Geometry: final body of the model. Coordinates: model frame, mm. Face numbers are marked on the shaded views. A direction names the side the tool comes from. Coordinates: 2 decimals unless noted, no trailing zeros. Loops run counter-clockwise (first coordinate to the right, second up) from the corner with the lowest first, then second, coordinate; pieces in that order, holes last. Notation, with made-up numbers: (-20.75, -33) -> (2.25, -33) arc R21 cw to (2.25, -11) -> close; hole circle Ø2 at (52.25, 50.5). An arc over 180 degrees is marked (long way). One line per item, written item: value. Start each with the question number.
from build123d import *

# Parameters (mm, degrees)
BOSS_EXTRUDE1_DEPTH     = 9
SKETCH2_W               = 152.4
SKETCH2_H               = 121
BOSS_EXTRUDE2_DEPTH     = 65
CHAMFER1_SIZE           = 10
SKETCH3_W               = 53.3
SKETCH3_H               = 12.5
CUT_EXTRUDE1_DEPTH      = 170.573612334
SKETCH4_R               = 2.5
BOSS_EXTRUDE3_DEPTH     = 1.780724539
CUT_EXTRUDE4_DEPTH      = 3
CUT_EXTRUDE4_DEPTH_BACK = 3
SKETCH5_R               = 1.5
CUT_EXTRUDE6_DEPTH      = 3
CUT_EXTRUDE6_DEPTH_BACK = 3
SKETCH7_W               = 9
SKETCH7_H               = 16.5
SKETCH8_R               = 8.25
CUT_EXTRUDE7_DEPTH      = 3
SKETCH9_R               = 1.5
CUT_EXTRUDE8_DEPTH      = 20


with BuildPart() as part:
    # Sketch1 → Boss-Extrude1 (new body)
    with BuildSketch(Plane(origin=(0, 0, 0), x_dir=(1, 0, 0), z_dir=(0, 1, 0))):
        with BuildLine():
            Line((-76.2, 63.5), (76.2, 63.5))
            ThreePointArc((76.2, 63.5), (85.180256121, 59.780256121), (88.9, 50.8))
            Line((88.9, 50.8), (88.9, -50.8))
            ThreePointArc((88.9, -50.8), (85.180256121, -59.780256121), (76.2, -63.5))
            Line((76.2, -63.5), (-76.2, -63.5))
            ThreePointArc((-76.2, -63.5), (-85.180256121, -59.780256121), (-88.9, -50.8))
            Line((-88.9, -50.8), (-88.9, 50.8))
            ThreePointArc((-88.9, 50.8), (-85.180256121, 59.780256121), (-76.2, 63.5))
        make_face()
    extrude(amount=BOSS_EXTRUDE1_DEPTH)

    # Sketch2 → Boss-Extrude2 (add)
    with BuildSketch(Plane(origin=(0, 9, 0), x_dir=(1, 0, 0), z_dir=(0, 1, 0))):
        with BuildLine():
            Line((76.2, 63.5), (-76.2, 63.5))
            ThreePointArc((-76.2, 63.5), (-85.180256121, 59.780256121), (-88.9, 50.8))
            Line((-88.9, 50.8), (-88.9, -50.8))
            ThreePointArc((-88.9, -50.8), (-85.180256121, -59.780256121), (-76.2, -63.5))
            Line((-76.2, -63.5), (76.2, -63.5))
            ThreePointArc((76.2, -63.5), (85.180256121, -59.780256121), (88.9, -50.8))
            Line((88.9, -50.8), (88.9, 50.8))
            ThreePointArc((88.9, 50.8), (85.180256121, 59.780256121), (76.2, 63.5))
        make_face()
        Rectangle(SKETCH2_W, SKETCH2_H, mode=Mode.SUBTRACT)
    extrude(amount=BOSS_EXTRUDE2_DEPTH)

    # Chamfer1
    chamfer1_edges = [part.edges().sort_by_distance(p)[0] for p in [
        (76.2, 41.5, -60.5),
        (-76.2, 41.5, -60.5),
        (-76.2, 41.5, 60.5),
        (76.2, 41.5, 60.5),
    ]]
    chamfer(chamfer1_edges, length=CHAMFER1_SIZE)

    # Sketch3 → Cut-Extrude1 (cut, through all)
    with BuildSketch(Plane.XY.offset(-60.5)):
        with Locations((-31.872362203, 17.030724539)):
            Rectangle(SKETCH3_W, SKETCH3_H)
    extrude(amount=-CUT_EXTRUDE1_DEPTH, mode=Mode.SUBTRACT)

    # Sketch4 → Boss-Extrude3 (add)
    with BuildSketch(Plane(origin=(0, 9, 0), x_dir=(1, 0, 0), z_dir=(0, 1, 0))):
        with Locations(Location((-56.511501143, 46.5, 0), (0, 0, 90))):
            Circle(SKETCH4_R)
        with Locations(Location((-8.211501143, 45.2, 0), (0, 0, 90))):
            Circle(SKETCH4_R)
        with Locations(Location((-23.411501143, -5.6, 0), (0, 0, 90))):
            Circle(SKETCH4_R)
        with Locations(Location((-51.311501143, -5.6, 0), (0, 0, 90))):
            Circle(SKETCH4_R)
    extrude(amount=BOSS_EXTRUDE3_DEPTH)

    # Sketch5 → Cut-Extrude4 (cut, two sides: drawn at the far end of the back side and taken through both)
    with BuildSketch(Plane(origin=(0, 10.780724539, 0), x_dir=(1, 0, 0), z_dir=(0, 1, 0)).offset(-CUT_EXTRUDE4_DEPTH_BACK)):
        with Locations(Location((-23.411501143, -5.6, 0), (0, 0, 270))):
            Circle(SKETCH5_R)
        with Locations(Location((-51.311501143, -5.6, 0), (0, 0, 270))):
            Circle(SKETCH5_R)
        with Locations(Location((-56.511501143, 46.5, 0), (0, 0, 270))):
            Circle(SKETCH5_R)
        with Locations(Location((-8.211501143, 45.2, 0), (0, 0, 270))):
            Circle(SKETCH5_R)
    extrude(amount=CUT_EXTRUDE4_DEPTH + CUT_EXTRUDE4_DEPTH_BACK, mode=Mode.SUBTRACT)

    # Sketch7 → Cut-Extrude6 (cut, two sides: drawn at the far end of the back side and taken through both)
    with BuildSketch(Plane.XY.offset(-60.5).offset(-CUT_EXTRUDE6_DEPTH_BACK)):
        with Locations((2.277637797, 19.030724539)):
            Rectangle(SKETCH7_W, SKETCH7_H)
    extrude(amount=CUT_EXTRUDE6_DEPTH + CUT_EXTRUDE6_DEPTH_BACK, mode=Mode.SUBTRACT)

    # Sketch8 → Cut-Extrude7 (cut)
    with BuildSketch(Plane.XY.offset(63.5)):
        with Locations((0, 37)):
            Circle(SKETCH8_R)
    extrude(amount=-CUT_EXTRUDE7_DEPTH, mode=Mode.SUBTRACT)

    # Sketch9 → Cut-Extrude8 (cut)
    with BuildSketch(Plane(origin=(0, 74, 0), x_dir=(1, 0, 0), z_dir=(0, 1, 0))):
        with Locations(Location((-80.555777772, -55.155777772, 0), (0, 0, 270))):
            Circle(SKETCH9_R)
        with Locations(Location((-80.555777772, 55.155777772, 0), (0, 0, 90))):
            Circle(SKETCH9_R)
        with Locations((29.755777772, -55.155777772)):
            Circle(SKETCH9_R)
        with Locations(Location((80.555777772, 55.155777772, 0), (0, 0, 270))):
            Circle(SKETCH9_R)
        with Locations(Location((80.555777772, -55.155777772, 0), (0, 0, 90))):
            Circle(SKETCH9_R)
    extrude(amount=-CUT_EXTRUDE8_DEPTH, mode=Mode.SUBTRACT)


solid = part.part
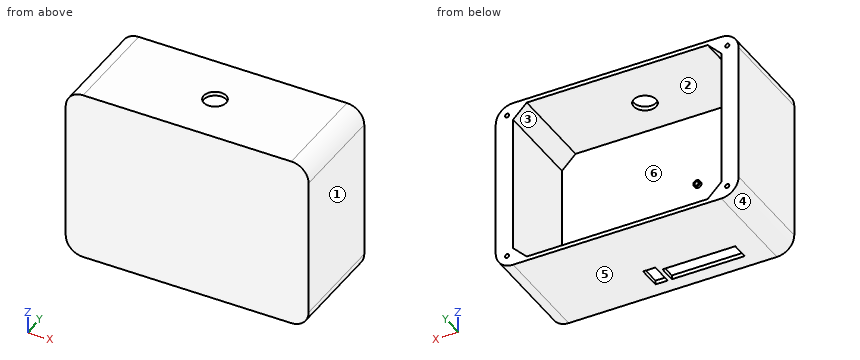
1. Line query: L1, parallel to X at y = 9.1, z = 5.6; L2, parallel to Z at x = 7, y = 58.5; L3, parallel to X at y = 38, z = 40. Output: solid intervals per line, ascending. Write a range as [from, to].
2. Section A-A on x = -40. Return the cut outline in (y, z), plus the area to 3 significant figures.
3. Draft query along X for the marked faces 3, 4, 5 and 6. Return one class per face: released by +X, released by -X, zero draft, split by the parting line, or undercut.
4. Set-up query: the marked faces 1 and 2. Return all of +Z, -Z, +X, -X, +Y, -Y with unobstructed straight access to the full face (end or side cutting, diameter ignored); none if empty.
5. Section C-C on y = 37. Return the cut outline in (x, z), plus the area to 3 significant figures.
6. Section B-B on x = 0. Return the cut outline in (y, z), plus the area to 3 significant figures.
7. Section D-D on z = -22.5. Return the cut outline in (x, y), plus the area to 3 significant figures.
8. Pin query (flat end, axial travel): pin 1 Ø2.5 at (y, z) = (18.5, -62.5) entering from +X; pin 2 Ø3.5 at (x, z) = (80, -55.5) entering from +Y; pin 3 Ø2.5 at (x, z) = (-23.41, 5.6) entering from +Y; pin 4 Ø3 at (x, z) = (59.5, 2.5) entering from +Y. Return the tip coordinate at first contact, or that it passes through.
Checks:
1. L1: [-88.9, -76.2], [-53.81, -52.81], [-49.81, -48.81], [-25.91, -24.91], [-21.91, -20.91], [76.2, 88.9]
1. L2: [-63.5, -60.5], [60.5, 63.5]
1. L3: [-88.9, -76.2], [76.2, 88.9]
2. outline: (0, -63.5) -> (10.78, -63.5) -> (10.78, -60.5) -> (9, -60.5) -> (9, 60.5) -> (74, 60.5) -> (74, 63.5) -> (0, 63.5) -> close; (23.28, -63.5) -> (74, -63.5) -> (74, -60.5) -> (23.28, -60.5) -> close
2. area: 1,500 mm²
3. face 3: undercut
3. face 4: released by -X
3. face 5: zero draft
3. face 6: undercut
4. face 1: +Z, -Z, +X, +Y, -Y
4. face 2: +Y
5. outline: (-88.9, -50.8) arc R12.7 ccw to (-76.2, -63.5) -> (76.2, -63.5) arc R12.7 ccw to (88.9, -50.8) -> (88.9, 50.8) arc R12.7 ccw to (76.2, 63.5) -> (8.25, 63.5) -> (8.25, 60.5) -> (66.2, 60.5) -> (76.2, 50.5) -> (76.2, -50.5) -> (66.2, -60.5) -> (-66.2, -60.5) -> (-76.2, -50.5) -> (-76.2, 50.5) -> (-66.2, 60.5) -> (-8.25, 60.5) -> (-8.25, 63.5) -> (-76.2, 63.5) arc R12.7 ccw to (-88.9, 50.8) -> close
5. area: 4,150 mm²
6. outline: (0, -63.5) -> (10.78, -63.5) -> (10.78, -60.5) -> (9, -60.5) -> (9, 60.5) -> (28.75, 60.5) -> (28.75, 63.5) -> (0, 63.5) -> close; (27.28, -63.5) -> (74, -63.5) -> (74, -60.5) -> (27.28, -60.5) -> close; (45.25, 60.5) -> (74, 60.5) -> (74, 63.5) -> (45.25, 63.5) -> close
6. area: 1,430 mm²
7. outline: (-88.9, 0) -> (88.9, 0) -> (88.9, 74) -> (76.2, 74) -> (76.2, 9) -> (-76.2, 9) -> (-76.2, 74) -> (-88.9, 74) -> close
7. area: 3,250 mm²
8. pin 1: x = 83.42
8. pin 2: y = 74
8. pin 3: y = 7.78
8. pin 4: y = 9
